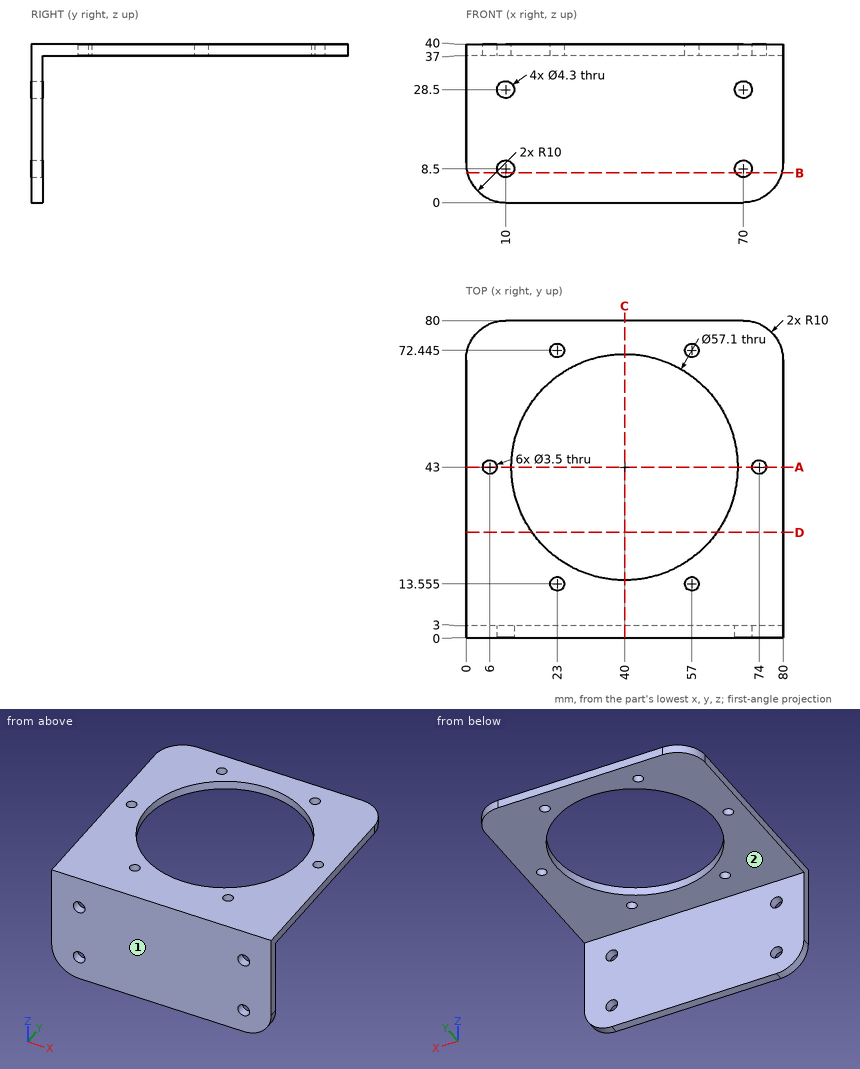
Input: dimensioned drawing with shaded views. Units: mm. Origin: part minimum x, y, z. A direction names the side the tool comes from. Give positions to 0.01 mm unless a question says otherwise; leave off trailing zeros. Loops run counter-clockwise (first coordinate to the right, second up) from the corner with the lowest first, then second, coordinate; pieces in that order, holes last. Notation, with made-up numbers: (34.25, 86) -> (92.25, 86) arc R19 ccw to (92.25, 118) -> close; hole circle Ø1 at (12.5, 20.5). An arc over 180 degrees is marked (long way). Use a Markdown table: item, result. Add a question column.
1) Reachability of the marked faces 1 and 2 from +Z, -Z, +X, -X, +Y, -Y: full face, straight path, thin tool, end or side. Return the list, or none.
2) Section query C-C, the plane x = 40. Return the cut outline in (y, z).
3) Section query D-D, the plane y = 26.5. Return the cut outline in (x, z).
4) Line query: line 1 along X through (y, z) = (2.45, 28.5); line 2 along Z through (x, y) = (10, 1); line 3 along Y through (x, z) = (4, 30.5). Output: solid intervals per line, ascending. Write a range as [from, to].
5) Section query A-A, the plane y = 43. Return the cut outline in (x, z).
6) Section query B-B, the plane z = 7.5. Return the cut outline in (x, y), then the cut area to 3 significant figures.
7) First-contact query: pin 1 (5.5 mm diameter, centred on x = 70, z = 8.5, fed in from +Y); pin 2 (4.5 mm diameter, centred on x = 74, y = 43, fed in from -Z). Flat tips, straight axial feed; report the tip coordinate or a pass-through.
Numbers:
| question | item | result |
|---|---|---|
| 1 | face 1 | +Z, -Z, +X, -X, -Y |
| 1 | face 2 | -Z, +X, -X, +Y |
| 2 | outline | (0, 0) -> (3, 0) -> (3, 37) -> (14.45, 37) -> (14.45, 40) -> (0, 40) -> close; (71.55, 37) -> (80, 37) -> (80, 40) -> (71.55, 40) -> close |
| 3 | outline | (0, 37) -> (16.7, 37) -> (16.7, 40) -> (0, 40) -> close; (63.3, 37) -> (80, 37) -> (80, 40) -> (63.3, 40) -> close |
| 4 | line 1 | x = [0, 7.85], [12.15, 67.85], [72.15, 80] |
| 4 | line 2 | z = [0, 6.35], [10.65, 26.35], [30.65, 40] |
| 4 | line 3 | y = [0, 3] |
| 5 | outline | (0, 37) -> (4.25, 37) -> (4.25, 40) -> (0, 40) -> close; (7.75, 37) -> (11.45, 37) -> (11.45, 40) -> (7.75, 40) -> close; (68.55, 37) -> (72.25, 37) -> (72.25, 40) -> (68.55, 40) -> close; (75.75, 37) -> (80, 37) -> (80, 40) -> (75.75, 40) -> close |
| 6 | outline | (0.32, 0) -> (8.1, 0) -> (8.1, 3) -> (0.32, 3) -> close; (11.9, 0) -> (68.1, 0) -> (68.1, 3) -> (11.9, 3) -> close; (71.9, 0) -> (79.68, 0) -> (79.68, 3) -> (71.9, 3) -> close |
| 6 | area | 215 mm2 |
| 7 | pin 1 | stops at y = 3 |
| 7 | pin 2 | stops at z = 37 |
